```python
from build123d import *

# Parameters (mm, degrees)
EXTRUDE_1_DEPTH = 30
SCALE_1_SCALE   = 1.7


with BuildPart() as part:
    # 草图1 → 凸台-拉伸1 (new body)
    with BuildSketch(Plane.XY):
        with BuildLine():
            Line((111.300105962, 44.956400142), (126.300105962, 29.956400142))
            Line((126.300105962, 29.956400142), (191.300105962, 29.956400142))
            ThreePointArc((191.300105962, 29.956400142), (206.300105962, 14.956400142), (191.300105962, -0.043599858))
            Line((191.300105962, -0.043599858), (-208.699894038, -0.043599858))
            Line((-208.699894038, -0.043599858), (-193.699894038, -15.043599858))
            Line((-193.699894038, -15.043599858), (191.300105962, -15.043599858))
            ThreePointArc((191.300105962, -15.043599858), (221.300105962, 14.956400142), (191.300105962, 44.956400142))
            Line((191.300105962, 44.956400142), (111.300105962, 44.956400142))
        make_face()
    extrude(amount=-EXTRUDE_1_DEPTH)


with BuildPart() as part_1:
    # 缩放比例1: scaled about (0, 0, 0)
    add(part.part.scale(SCALE_1_SCALE))


solid = part_1.part
```
Source: CAD feature listing. Evaluate the final solid. Frame: model axes, mm. A direction names the side the tool comes from. Coordinates: 2 decimals unless noted, no trailing zeros. Loops run counter-clockwise (first coordinate to the right, second up) from the corner with the lowest first, then second, coordinate; pieces in that order, holes last. Notation, with made-up numbers: M 16.5,13.5 L 68.5,13.5 A11 ccw 68.5,24.5 Z; hole C -13.5,6 d10. An arc over 180 degrees is marked long. Put each result on its own line as item: value. Start each with the question number.
1) Cut plane A-A on x = 232. Return the cut outline in (y, z).
2) Contact query for flat-ended pins moving along their axis: pin 1 Ø2 at (y, z) = (18, -42.5) entering from -X; pin 2 Ø6 at (y, z) = (12, -34) entering from -X; pin 3 Ø1.5 at (x, z) = (-170.5, -35) entering from +Y. Output: stop coordinate, or through.
3) Cut plane C-C on y = -13.5. Return the cut outline in (x, z), then the cut area to 3 significant figures.
4) Cut plane D-D on x = -274. Return the cut outline in (y, z).
5) Pull-direction query (Y, two-part tool) for faces 1 (the face through (201.782, 63.854, -25.143)), 2 (the face through (63, -1, -51)), 3 (the face through (258, 76.426, -25)); classes: pulls with the +Y half, pulls with the -Y half, needs draft (parallel to the pull), parting line crosses it, or undercut.
6) Cut plane B-B on z = -9.5. Return the cut outline in (x, y).
7) Ray query, L1, parallel to Y at x = 66, z = -15; L2, parallel to X at y = 14, z = -40.5; L3, parallel to X at y = 6, z = -30. Return the intervals inside material, ascending. Write a range as from..to.
8) Reachability of faces 4 (the face through (-7, -25.574, -25)), 5 (the face through (-10, -0.074, -25)) from +Z, -Z, +X, -X, +Y, -Y: full face, straight path, thin tool, end or side. Return the list, or none.
The answers:
1. outline: M -25.57,-51 L -0.07,-51 L -0.07,0 L -25.57,0 Z; M 50.93,-51 L 76.43,-51 L 76.43,0 L 50.93,0 Z
2. pin 1: stops at x = 349.28
2. pin 2: stops at x = 344.72
2. pin 3: stops at y = -0.07
3. outline: M -341.36,-51 L 358.16,-51 L 358.16,0 L -341.36,0 Z
3. area: 35,700 mm²
4. outline: M -25.57,-51 L -0.07,-51 L -0.07,0 L -25.57,0 Z
5. face 1: undercut
5. face 2: needs draft
5. face 3: pulls with the +Y half
6. outline: M -354.79,-0.07 L -329.29,-25.57 L 325.21,-25.57 A51 ccw 325.21,76.43 L 189.21,76.43 L 214.71,50.93 L 325.21,50.93 A25.5 cw 325.21,-0.07 Z
7. L1: y = -25.57..-0.07
7. L2: x = 348.01..374.91
7. L3: x = 341.73..372.37
8. face 4: +Z, -Z, +X, -X, -Y
8. face 5: +Z, -Z, -X
